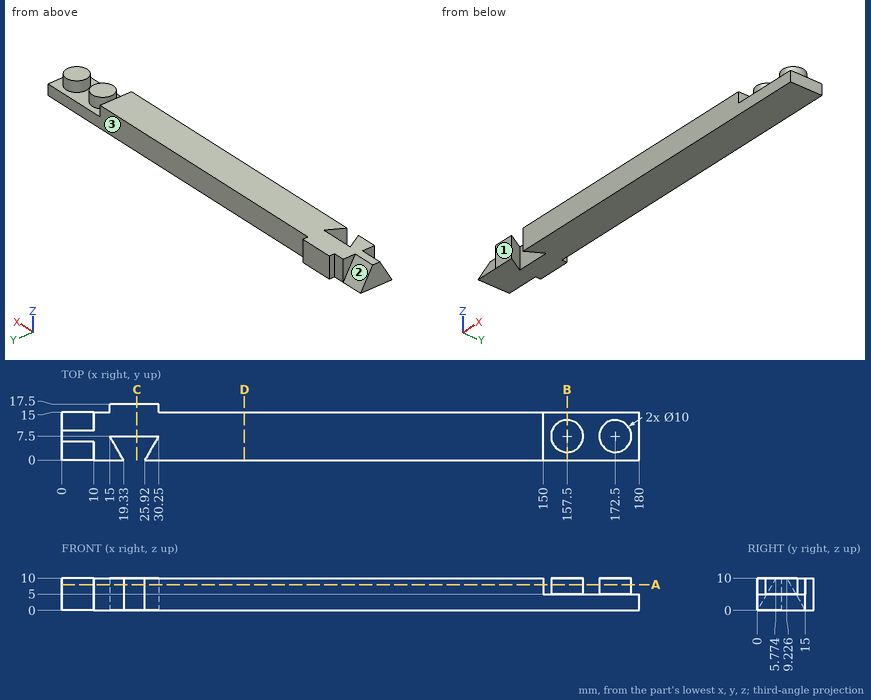
Source: three-view drawing plus pictorial views. Frame: mm from the lowest corner of the part. A direction names the side the tool comes from. Coordinates: 2 decimals unless noted, no trailing zeros. Order: outer loops, then holes, each group sorted by start corner. A loop starts at its lowest first (then second) coordinate and runs counter-clockwise, first axis right, second up. Notation, with made-up numbers: M -19.5,36.25 L 9.5,36.25 A22 ccw 9.5,74.25 Z; hole C 88.25,64 d9. An arc over 180 degrees is marked long. Write each question's results on one line, items separated by ' | '. Start each with the question number.
1. Section C-C, the plane x = 23.5. Return the cut outline in (y, z), then the cut area to 3 significant figures.
2. Section B-B, the plane x = 157.5. Return the cut outline in (y, z).
3. Section D-D, the plane x = 57. Return the cut outline in (y, z).
4. Reachability of the marked faces 1, 2 and 3 from +Z, -Z, +X, -X, +Y, -Y: full face, straight path, thin tool, end or side. Return the list, or none.
5. Pin query (flat end, axial travel): pin 1 (2 mm diameter, centred on y = 5, z = 7.5, fed in from +X); pin 2 (4 mm diameter, centred on x = 11.5, z = 4, fed in from +Y); pin 3 (1.5 mm diameter, centred on y = 6.5, z = 8, fed in from +X); pin 4 (5 mm diameter, centred on y = 7, z = 7.5, fed in from -X). Return the tip coordinate at first contact, or that it passes through.
6. Section A-A, the plane z = 8. Return the cut outline in (x, y).
7. Material intervals for L1, parallel to Y at x = 158, z = 7 (1 decimal); L2, parallel to X at y = 14.5, z = 9.75; L3, parallel to X at y = 9.75, z = 8.25 (1 decimal), sorted ascending.
Solution:
1) outline: M 7.5,0 L 17.5,0 L 17.5,10 L 7.5,10 Z | area: 100 mm²
2) outline: M 0,0 L 15,0 L 15,5 L 12.5,5 L 12.5,10 L 2.5,10 L 2.5,5 L 0,5 Z
3) outline: M 0,0 L 15,0 L 15,10 L 0,10 Z
4) face 1: +Z, -Z, +X, -X, -Y | face 2: +Z, -X, +Y | face 3: +Z, -Z, +X, +Y
5) pin 1: x = 177.27 | pin 2: y = 15 | pin 3: x = 177.49 | pin 4: x = 0
6) outline: M 0,4.62 L 10,4.62 L 10,0 L 19.33,0 L 15,7.5 L 30.25,7.5 L 25.92,0 L 150,0 L 150,15 L 30.25,15 L 30.25,17.5 L 15,17.5 L 15,15 L 10,15 L 10,10.38 L 0,10.38 Z; C 157.5,7.5 d10; C 172.5,7.5 d10
7) L1: 2.5 to 12.5 | L2: 10 to 150 | L3: 0 to 150, 153 to 162, 168 to 177
